Check sheet for the modelled part. Datum: model origin and axes. Units: mm. A direction names the side the tool comes from. Round coordinates to 2 decimals unless told otherwise and drop trailing zeros. Write each loop counter-clockwise with the first axis right and the second up, starting at its lowest first coordinate (ties: lowest second). Pieces come first, ordered by that corner, then holes.
from build123d import *

# Parameters (mm, degrees)
F0_W      = 80
F0_H      = 7
F1_DEPTH  = 2
F0_H_2    = 2
F2_DEPTH  = 13
F3_W      = 1
F3_H      = 3
F4_DEPTH  = 80
F5_R      = 1
F6_R      = 1
F7_R      = 1.49999
F8_R      = 0.49999
F10_DEPTH = 0.5


# Not quite as in the source:
# - a fillet or chamfer is up to 0.001 mm smaller than in the source, because OpenCascade refuses the exact size
# - a feature names something its author has since deleted; it is built from what else it names


with BuildPart() as f1:
    # F0 (on Top) → F1 (new body)
    with BuildSketch(Plane.XY):
        Rectangle(F0_W, F0_H)
    extrude(amount=F1_DEPTH)

    # F0 (on Top) → F2 (join)
    with BuildSketch(Plane.XY):
        with Locations((0, 4.5)):
            Rectangle(F0_W, F0_H_2)
        with Locations((0, -4.5)):
            Rectangle(F0_W, F0_H_2)
    extrude(amount=F2_DEPTH)

    # F3 (on face) → F4 (join)
    with BuildSketch(Plane(origin=(-40, 0, 0), x_dir=(0, -1, 0), z_dir=(-1, 0, 0))):
        Polygon((-3.5, 13), (-3.5, 9), (-2.8, 11), align=None)
        Polygon((2.8, 11), (3.5, 9), (3.5, 13), align=None)
        with Locations((0, 3.5)):
            Rectangle(F3_W, F3_H)
    extrude(amount=-F4_DEPTH)

    # F5
    f5_edges = [f1.edges().sort_by_distance(p)[0] for p in [
        (0, 2.8, 11),
    ]]
    fillet(f5_edges, radius=F5_R)

    # F6
    f6_edges = [f1.edges().sort_by_distance(p)[0] for p in [
        (0, -2.8, 11),
    ]]
    fillet(f6_edges, radius=F6_R)

    # F7 (radius 1.5 in the source; OpenCascade refuses exactly that, so slightly less here)
    f7_edges = [f1.edges().sort_by_distance(p)[0] for p in [
        (0, -3.5, 2),
        (0, 3.5, 2),
        (0, -0.5, 2),
        (0, 0.5, 2),
    ]]
    fillet(f7_edges, radius=F7_R)

    # F8 (radius 0.5 in the source; OpenCascade refuses exactly that, so slightly less here)
    f8_edges = [f1.edges().sort_by_distance(p)[0] for p in [
        (0, -0.5, 5),
        (0, 0.5, 5),
        (-40, 0, 5),
        (40, 0, 5),
    ]]
    fillet(f8_edges, radius=F8_R)

    # F9 (on face) → F10 (join)
    with BuildSketch(Plane(origin=(0, 0, 0), x_dir=(1, 0, 0), z_dir=(0, 0, -1))):
        with BuildLine():
            ThreePointArc((-40, 2), (-42.7386127875, 1.4821200219), (-45.0990195136, 0))
            ThreePointArc((-45.0990195136, 0), (-42.7386127875, -1.4821200219), (-40, -2))
            Line((-40, -2), (-40, 2))
        make_face()
        with BuildLine():
            Line((-40, 5.5), (-32.5, 5.5))
            ThreePointArc((-32.5, 5.5), (-43.0006127414, 12.3735960876), (-45.0990195136, 0))
            ThreePointArc((-45.0990195136, 0), (-42.7386127875, 1.4821200219), (-40, 2))
            Line((-40, 2), (-40, 5.5))
        make_face()
        with BuildLine():
            ThreePointArc((-40, -2), (-42.7386127875, -1.4821200219), (-45.0990195136, 0))
            ThreePointArc((-45.0990195136, 0), (-43.0006127414, -12.3735960876), (-32.5, -5.5))
            Line((-32.5, -5.5), (-40, -5.5))
            Line((-40, -5.5), (-40, -2))
        make_face()
        with BuildLine():
            Line((40, -5.5), (32.5, -5.5))
            ThreePointArc((32.5, -5.5), (40, -13), (47.5, -5.5))
            ThreePointArc((47.5, -5.5), (46.8735960876, -2.4993872586), (45.0990195136, 0))
            ThreePointArc((45.0990195136, 0), (42.7386127875, -1.4821200219), (40, -2))
            Line((40, -2), (40, -5.5))
        make_face()
        with BuildLine():
            ThreePointArc((40, -2), (42.7386127875, -1.4821200219), (45.0990195136, 0))
            ThreePointArc((45.0990195136, 0), (42.7386127875, 1.4821200219), (40, 2))
            Line((40, 2), (40, -2))
        make_face()
        with BuildLine():
            ThreePointArc((47.5, 5.5), (40, 13), (32.5, 5.5))
            Line((32.5, 5.5), (40, 5.5))
            Line((40, 5.5), (40, 2))
            ThreePointArc((40, 2), (42.7386127875, 1.4821200219), (45.0990195136, 0))
            ThreePointArc((45.0990195136, 0), (46.8735960876, 2.4993872586), (47.5, 5.5))
        make_face()
    extrude(amount=-F10_DEPTH)


solid = f1.part
1. Scan lines: line 1 along Y through (x, z) = (10.5, 7); line 2 along Y through (x, z) = (37.5, 3.5); line 3 along Y through (x, z) = (18, 2.5). Record each from-to range of solid material in increasing order.
2. Go/stop test with flat-tipped pins: pin 1 (4 mm diameter, centred on x = 17, z = 3.5, fed in from +Y); pin 2 (5.5 mm diameter, centred on y = -1, z = 8.5, fed in from -X); pin 3 (1.5 mm diameter, centred on x = -33, z = 8, fed in from -Y). Record where each tip stops, or that it passes through.
3. Set-up check for faces 1 (the flat face through (40, 0, 4)), 2 (the cylindrical face through (0.56, 0.93, 2.45)), 3 (the flat face through (-0.56, 3.212, 9.823)): record each of +Z, -Z, +X, -X, +Y, -Y from which the full face is reachable in a straight line by a thin tool's end or side.
4. Release check for a two-part mould opening along Y. For faces 4 (the flat face through (-0.56, -3.204, 9.847)), 5 (the flat face through (-0.56, 3.204, 12.153)), 6 (the flat face through (-1, -5.5, 6)), 7 (the flat face through (-1, -4, 13)) record: released by +Y, released by -Y, zero draft, split by the parting line, or undercut.
5. Sectioned sample at A-A, the plane y = -7. Enter the section's corners in (x, z).
Computed values:
1. line 1: y = -5.5 to -3.5, 3.5 to 5.5
1. line 2: y = -5.5 to -3.5, -0.5 to 0.5, 3.5 to 5.5
1. line 3: y = -5.5 to -3.12, -0.88 to 0.88, 3.12 to 5.5
2. pin 1: stops at y = 5.5
2. pin 2: stops at x = -40
2. pin 3: stops at y = -5.5
3. face 1: +Z, +X, +Y, -Y
3. face 2: +Z, +X, -X
3. face 3: +X, -X
4. face 4: undercut
4. face 5: undercut
4. face 6: released by -Y
4. face 7: zero draft
5. outline: (-47.35, 0) - (-32.65, 0) - (-32.65, 0.5) - (-47.35, 0.5) - close; (32.65, 0) - (47.35, 0) - (47.35, 0.5) - (32.65, 0.5) - close
